Verification items for this drawing (mm, ordinates from the low corner). A direction names the side the tool comes from. Round coordinates to 2 decimals unless told otherwise and drop trailing zeros. Loops run counter-clockwise (first coordinate to the right, second up) from the corner with the lowest first, then second, coordinate; pieces in that order, holes last. Notation, with made-up numbers: (74, 68.25) -> (97, 68.25) arc R15 cw to (97, 80.25) -> close; hole circle Ø10 at (20.25, -21). An arc over 180 degrees is marked (long way). Use a Markdown table: item, result. Add a question column.
Q1. Sectioned sample at A-A, the plane z = 34. Enter the section's corners in (x, y), then the cut area to 3 significant figures.
Q2. Release check for a two-part mould opening along X. For the marked faces 4, 5, 6 and 7 record: released by +X, released by -X, zero draft, split by the parting line, or undercut.
Q3. Set-up check for the marked faces 1, 2 and 3: record each of +Z, -Z, +X, -X, +Y, -Y from which the full face is reachable in a straight line by a thin tool's end or side.
Q4. Material ranges on L1, parallel to X at y = 4, z = 36; L2, parallel to Y at x = 1.25, z = 44; L3, parallel to X at y = 22.5, z = 36, recorded low to high.
Q5. Sectioned sample at D-D, the plane y = 6. Enter the section's corners in (x, z).
Q6. Gauge pin test, flat ends, axial feed: P1, Ø1.5, axis at x = 31.5, y = 21.5, coming from the +Z side; P2, Ø6.5, axis at y = 20, z = 44, coming from the +X side; P3, Ø3, axis at y = 7, z = 34.5, coming from the -X side. Record the tip position at first contact, or that the pin passes through.
Q7. Sectioned sample at C-C, the plane y = 30. Enter the section's corners in (x, z) (3 decimals), then the cut area to 3 significant figures.
Q8. Sectioned sample at B-B, the plane y = 20. Enter the section's corners in (x, z).
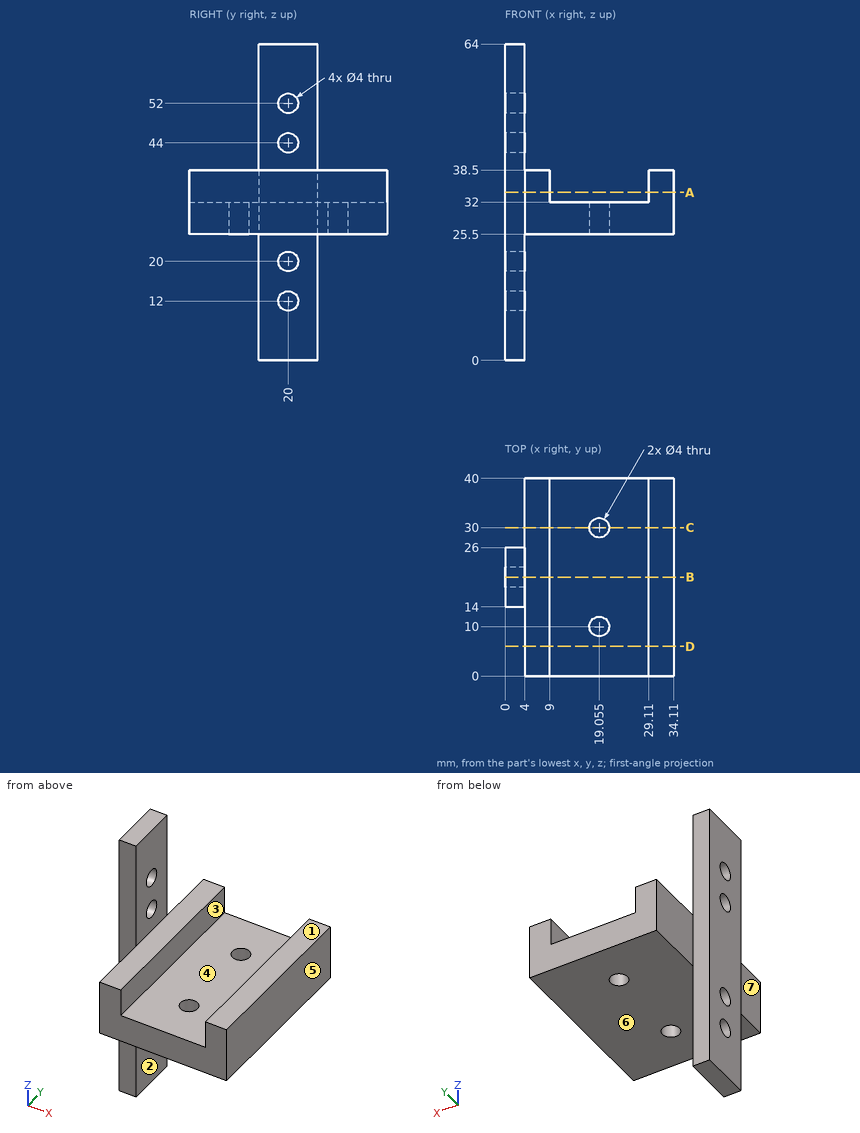
Values:
| question | item | result |
|---|---|---|
| 1 | outline | (0, 14) -> (4, 14) -> (4, 0) -> (9, 0) -> (9, 40) -> (4, 40) -> (4, 26) -> (0, 26) -> close; (29.11, 0) -> (34.11, 0) -> (34.11, 40) -> (29.11, 40) -> close |
| 1 | area | 448 mm^2 |
| 2 | face 4 | undercut |
| 2 | face 5 | released by +X |
| 2 | face 6 | zero draft |
| 2 | face 7 | released by -X |
| 3 | face 1 | +Z, +X, +Y, -Y |
| 3 | face 2 | -Z, +X, +Y, -Y |
| 3 | face 3 | +Z, +Y, -Y |
| 4 | L1 | 4 to 9, 29.11 to 34.11 |
| 4 | L2 | 14 to 18, 22 to 26 |
| 4 | L3 | 0 to 9, 29.11 to 34.11 |
| 5 | outline | (4, 25.5) -> (34.11, 25.5) -> (34.11, 38.5) -> (29.11, 38.5) -> (29.11, 32) -> (9, 32) -> (9, 38.5) -> (4, 38.5) -> close |
| 6 | P1 | z = 38.5 |
| 6 | P2 | x = 4 |
| 6 | P3 | x = 4 |
| 7 | outline | (4, 25.5) -> (17.055, 25.5) -> (17.055, 32) -> (9, 32) -> (9, 38.5) -> (4, 38.5) -> close; (21.055, 25.5) -> (34.11, 25.5) -> (34.11, 38.5) -> (29.11, 38.5) -> (29.11, 32) -> (21.055, 32) -> close |
| 7 | area | 235 mm^2 |
| 8 | outline | (0, 0) -> (4, 0) -> (4, 10) -> (0, 10) -> close; (0, 14) -> (4, 14) -> (4, 18) -> (0, 18) -> close; (0, 22) -> (4, 22) -> (4, 25.5) -> (34.11, 25.5) -> (34.11, 38.5) -> (29.11, 38.5) -> (29.11, 32) -> (9, 32) -> (9, 38.5) -> (4, 38.5) -> (4, 42) -> (0, 42) -> close; (0, 46) -> (4, 46) -> (4, 50) -> (0, 50) -> close; (0, 54) -> (4, 54) -> (4, 64) -> (0, 64) -> close |
